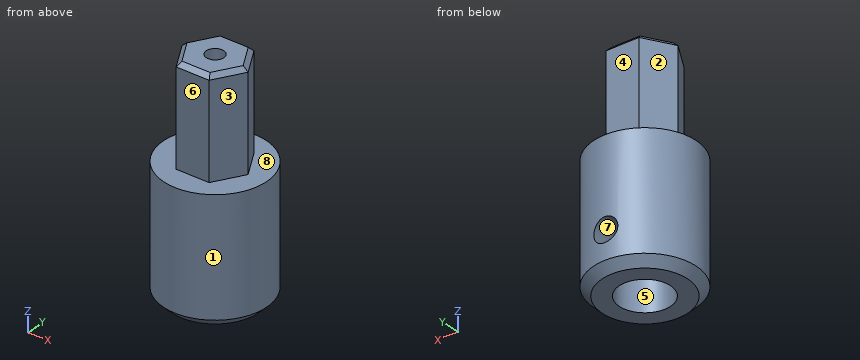
from build123d import *

# Parameters (mm, degrees)
SKETCH_1_R               = 6
EXTRUDE_1_DEPTH          = 14.5
EXTRUDE_2_DEPTH          = 11.5
HOLE_WIZARD_M2_5_1_D     = 2.05
HOLE_WIZARD_M2_5_1_DEPTH = 11
HOLE_WIZARD_M2_5_1_TIP   = 0.615882135
SKETCH_6_R               = 3
CUT_EXTRUDE_1_DEPTH      = 12
CHAMFER_2_SIZE           = 1
CHAMFER_3_SIZE           = 0.5
SKETCH_7_R               = 1.4
CUT_EXTRUDE_2_DEPTH      = 6


with BuildPart() as part:
    # 草图1 → 凸台-拉伸1 (new body)
    with BuildSketch(Plane.XY):
        with Locations(Location((0, 0, 0), (0, 0, 180))):
            Circle(SKETCH_1_R)
    extrude(amount=EXTRUDE_1_DEPTH)

    # 草图2 → 凸台-拉伸2 (add)
    with BuildSketch(Plane.XY.offset(14.5)):
        Polygon((3.868246804, 0), (1.934123402, 3.35), (-1.934123402, 3.35), (-3.868246804, 0), (-1.934123402, -3.35), (1.934123402, -3.35), align=None)
    extrude(amount=EXTRUDE_2_DEPTH)

    # M2.5 螺纹孔1
    with Locations(Plane.XY.offset(26)):
        with Locations((0, 0)):
            Hole(HOLE_WIZARD_M2_5_1_D / 2, depth=HOLE_WIZARD_M2_5_1_DEPTH)
            with Locations((0, 0, -(HOLE_WIZARD_M2_5_1_DEPTH + HOLE_WIZARD_M2_5_1_TIP / 2))):  # 118° drill point
                Cone(0, HOLE_WIZARD_M2_5_1_D / 2, HOLE_WIZARD_M2_5_1_TIP, mode=Mode.SUBTRACT)

    # 草图6 → 切除-拉伸1 (cut)
    with BuildSketch(Plane(origin=(0, 0, 0), x_dir=(-1, 0, 0), z_dir=(0, 0, -1))):
        Circle(SKETCH_6_R)
    extrude(amount=-CUT_EXTRUDE_1_DEPTH, mode=Mode.SUBTRACT)

    # 倒角2
    chamfer_2_edges = [part.edges().sort_by_distance(p)[0] for p in [
        (6, 0, 0),
    ]]
    chamfer(chamfer_2_edges, length=CHAMFER_2_SIZE)

    # 倒角3
    chamfer_3_edges = [part.edges().sort_by_distance(p)[0] for p in [
        (2.901185103, -1.675, 26),
        (2.901185103, 1.675, 26),
        (0, 3.35, 26),
        (-2.901185103, 1.675, 26),
        (-2.901185103, -1.675, 26),
        (0, -3.35, 26),
    ]]
    chamfer(chamfer_3_edges, length=CHAMFER_3_SIZE)

    # 草图7 → 切除-拉伸2 (cut)
    with BuildSketch(Plane(origin=(0, 6, 0), x_dir=(1, 0, 0), z_dir=(0, 1, 0))):
        with Locations(Location((0, -4.3, 0), (0, 0, 270))):
            Circle(SKETCH_7_R)
    extrude(amount=-CUT_EXTRUDE_2_DEPTH, mode=Mode.SUBTRACT)


solid = part.part
Could you check a few things on this model? Use its own coordinates, in mm. Face numbers are marked on the shaded views. A direction names the side the tool comes from. Coordinates: 2 decimals unless noted, no trailing zeros. Loops run counter-clockwise (first coordinate to the right, second up) from the corner with the lowest first, then second, coordinate; pieces in that order, holes last. Notation, with made-up numbers: (5.5, 33.25) -> (35.5, 33.25) arc R8 cw to (35.5, 47.25) -> close; hole circle Ø7 at (46, -30). An arc over 180 degrees is marked (long way). Answer in a Markdown table with one row per item.
(1) Imagine slicing it at A-A (z = 20.75). List the corners of the cut face in (x, y) for me (3 decimals), plus the area to 3 significant figures.
Results found:
| item | result |
|---|---|
| outline | (-3.868, 0) -> (-1.934, -3.35) -> (1.934, -3.35) -> (3.868, 0) -> (1.934, 3.35) -> (-1.934, 3.35) -> close; hole circle Ø2.05 at (0, 0) |
| area | 35.6 mm^2 |
(2) Imagine slicing it at B-B (z = 8.75). List the corners of the cut face in (x, y) for me.
Results found:
| item | result |
|---|---|
| outline | circle Ø12 at (0, 0); hole circle Ø6 at (0, 0) |
(3) Imagine slicing it at C-C (z = 4.3). List the corners of the cut face in (x, y) for me.
Results found:
| item | result |
|---|---|
| outline | (-1.4, 2.65) -> (-1.4, 5.83) arc R6 ccw (long way) to (1.4, 5.83) -> (1.4, 2.65) arc R3 cw (long way) to start |
(4) Thinking about a two-plate mould opening in Z: for the marked faces 6, 7 and 8, which applies, released by +Z, released by -Z, zero draft, split by the parting line, or undercut?
Results found:
| item | result |
|---|---|
| face 6 | zero draft |
| face 7 | undercut |
| face 8 | released by +Z |
(5) For the marked faces 1, 2, 3, 4 and 5, which set-ups out of +Z, -Z, +X, -X, +Y, -Y let a thin tool reach every point of the face, with its end or its side?
Results found:
| item | result |
|---|---|
| face 1 | +Z, -Z |
| face 2 | +Z, -X, +Y |
| face 3 | +Z, +X, -Y |
| face 4 | +Z, +X, -X, +Y |
| face 5 | -Z |
(6) If I drill on probe 1 along Y at (x, z) = (0, 22.5) (3 decimals); probe 2 along Z at (x, y) = (-1.75, -2.25); probe 3 along Z at (x, y) = (3.5, -1.5), over which ranges is the centre line in solid material (lowest first)?
Results found:
| item | result |
|---|---|
| probe 1 | y = -3.35 to -1.025, 1.025 to 3.35 |
| probe 2 | z = 12 to 26 |
| probe 3 | z = 0 to 14.5 |
(7) Will these pins go through, and if not, where does the flat tip stop? pin 1 Ø1.8 at (x, y) = (0, 0) entering from +Z; pin 2 Ø3.5 at (x, y) = (0, 0) entering from -Z; pin 3 Ø2 at (y, z) = (3, 6.5) entering from +X.
Results found:
| item | result |
|---|---|
| pin 1 | stops at z = 14.92 |
| pin 2 | stops at z = 12 |
| pin 3 | stops at x = 5.66 |
